Could you check a few things on this model? Use its own coordinates, in mm. Face numbers are marked on the shaded views. Round coordinates to 2 decimals unless told otherwise and drop trailing zeros. Write each loop counter-clockwise with the first axis right and the second up, starting at its lowest first coordinate (ties: lowest second). Pieces come first, ordered by that corner, then holes. Notation, with made-up numbers: (-19.75, 38.5) -> (-11.75, 38.5) arc R23 ccw to (-11.75, 71.5) -> close; hole circle Ø7 at (73, 87.25). An arc over 180 degrees is marked (long way). Answer in a Markdown table with one row per item. Add a question column.
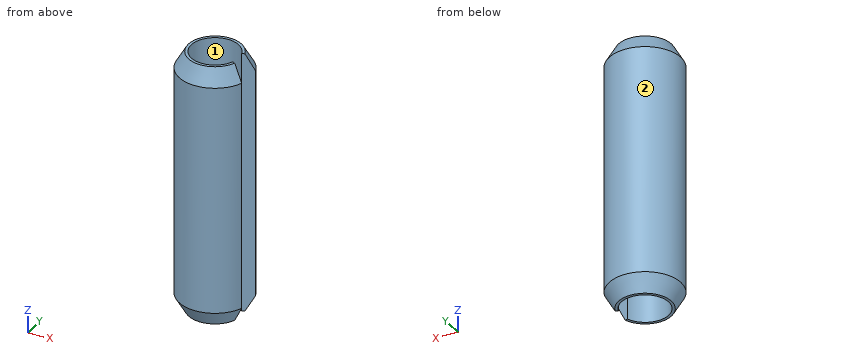
Autodesk Inventor part; units mm, degrees
ref_plane "YZ Plane" through (0, 0, 0) normal (1, 0, 0) x (0, 1, 0)
ref_plane "XZ Plane" through (0, 0, 0) normal (0, 1, 0) x (-1, 0, 0)
ref_plane "XY Plane" through (0, 0, 0) normal (0, 0, 1) x (1, 0, 0)
sketch "Sketch1" plane through (0, 0, 0) normal (0, 0, 1) x (1, 0, 0)
  arc A0 (2.0651, 0.7586) -> (2.0651, -0.7586) centre (0, 0) ccw
  arc A1 (1.3611, 0.5) -> (1.3611, -0.5) centre (0, 0) ccw
  line L0 (2.0651, 0.7586) -> (1.3611, 0.5)
  line L1 (0, 0) -> (1.3611, -0.5) construction
  line L2 (1.3611, 0.5) -> (0, 0) construction
  line L3 (1.3611, -0.5) -> (2.0651, -0.7586)
  line L4 (-3.053, 0) -> (2.9181, 0) construction
  dimension "d0" = 4.4
  dimension "d1" = 2.9
  dimension "d2" = 1
extrude "Extrusion1" add sketch "Sketch1" along normal mid plane 16
chamfer "Chamfer1" distance 1 angle 30 2 edges at (-2.2, 0, 8) (-2.2, 0, -8) measured on face at (-1.7005, -1.3958, -2.6667)
properties material "ABS Plastic"
(1) I need wall thicknesses on L1, parallel to Y at x = 0, z = 2.5; L2, parallel to Y at x = 1.75, z = -6.75; L3, parallel to X at y = 0.85, z = -5.75. Which ranges of each line are inside material? Lowest first, please.
(2) Suppose I cut it at B-B, the plane y = 0. Please give me the cut outline in (x, z).
(3) Suppose I cut it at A-A, the plane x = 0. Please give me the cut outline in (y, z), then the cut area to 3 significant figures.
(4) Suppose I cut it at C-C, the plane z = -4.5. Please give me the cut outline in (x, y).
(5) If we mould it in two halves opening along X, with no side actions, what happens to the marked faces 1 and 2? For each: pulls with the +X half, pulls with the -X half, needs draft (parallel to the pull), parting line crosses it, or undercut.
Response:
| question | item | result |
|---|---|---|
| 1 | L1 | -2.2 to -1.45, 1.45 to 2.2 |
| 1 | L2 | -1.33 to -0.64, 0.64 to 1.33 |
| 1 | L3 | -2.03 to -1.17, 1.17 to 2.03 |
| 2 | outline | (-2.2, -7) -> (-1.62, -8) -> (-1.45, -8) -> (-1.45, 8) -> (-1.62, 8) -> (-2.2, 7) -> close |
| 3 | outline | (-2.2, -7) -> (-1.62, -8) -> (-1.45, -8) -> (-1.45, 8) -> (-1.62, 8) -> (-2.2, 7) -> close; (1.45, -8) -> (1.62, -8) -> (2.2, -7) -> (2.2, 7) -> (1.62, 8) -> (1.45, 8) -> close |
| 3 | area | 22.8 mm² |
| 4 | outline | (1.36, -0.5) arc R1.45 cw (long way) to (1.36, 0.5) -> (2.07, 0.76) arc R2.2 ccw (long way) to (2.07, -0.76) -> close |
| 5 | face 1 | undercut |
| 5 | face 2 | parting line crosses it |
